Read the model definition and answer for the solid it produces. Units are mm, in the model's axes. A direction names the side the tool comes from. Coordinates: 2 decimals unless noted, no trailing zeros. Order: outer loops, then holes, each group sorted by start corner. A loop starts at its lowest first (then second) coordinate and runs counter-clockwise, first axis right, second up. Notation, with made-up numbers: (79.5, -5.5) -> (122.5, -5.5) arc R20 ccw to (122.5, 23.5) -> close; hole circle Ø7 at (-17.75, -12.75). An arc over 180 degrees is marked (long way). Answer as a JSON object with one key per item and string values. Group by question number.
1) A tool of negligible diameter and unlimited length cuts with its end or side. For faces 1 (the flat face through (-34, -4, 17.8)), 2 (the flat face through (-9, 66, 17.8)), 3 (the flat face through (18.9, 40, 17)), from which of +Z, -Z, +X, -X, +Y, -Y can it reach the whole face along a straight path? Write none if from no direction.
2) Section C-C on y = 53.5 is taken. Determine the outline of the cut face in (x, z).
3) Consider L1, parallel to X at y = 5, z = 16.8; L2, parallel to Y at x = -53, z = 18.5; L3, parallel to Y at x = -33, z = 18.7. Determine where each line is inside the solid, lowest interval first.
4) Section D-D on x = 46 is taken. Determine the outline of the cut face in (y, z), and give its area (3 significant figures).
5) Section B-B on x = -24.13 is taken. Determine the outline of the cut face in (y, z), and give its area (3 significant figures).
6) Determine the mould class of faces 4 (the flat face through (14.53, 37.6, 17.48)), 5 (the flat face through (25, 65, 17)) for opening direction X: released by +X, released by -X, zero draft, split by the parting line, or undercut.
7) Given pin 1 (1.5 mm diameter, centred on x = -23, y = 11.5, fed in from -Z); pin 2 (0.9 mm diameter, centred on y = 40.5, z = 17.5, fed in from -X); pin 3 (1.4 mm diameter, centred on x = 33, y = -3, fed in from -Z); pin 4 (1.5 mm diameter, centred on x = 20.5, z = 18, fed in from +Y), each flat-ended and moving along its own axis, determine where each tip first touches the part or whether it passes through.
8) Section A-A on x = 2.7 is taken. Determine the outline of the cut face in (y, z), and give its area (3 significant figures).
from build123d import *

# Parameters (mm, degrees)
PAD001_DEPTH         = 3
SKETCH012_R          = 1.4
POCKET005_DEPTH      = 3.001
SKETCH014_R          = 2.5
POCKET006_DEPTH      = 1.8
POCKET008_DEPTH      = 0.001
POCKET008_DEPTH_BACK = 3.001
SKETCH017_R          = 1.15
POCKET009_DEPTH      = 0.001
POCKET009_DEPTH_BACK = 3.001
POCKET010_DEPTH      = 1.8
SKETCH023_R          = 1.15
POCKET013_DEPTH      = 0.001
POCKET013_DEPTH_BACK = 3.001
SKETCH026_R          = 2.15
POCKET016_DEPTH      = 2.001


with BuildPart() as part:
    # Sketch009 → Pad001 (new body)
    with BuildSketch(Plane.XY):
        with BuildLine():
            Line((56.5, 38), (56.5, -1))
            ThreePointArc((54.5, -3), (55.914214, -2.414214), (56.5, -1))
            Line((54.5, -3), (30.5, -3))
            ThreePointArc((29.5, -2), (29.792893, -2.707107), (30.5, -3))
            Line((29.5, -2), (29.5, -1))
            ThreePointArc((29.5, -1), (29.207107, -0.292893), (28.5, 0))
            Line((28.5, 0), (-28.5, 0))
            ThreePointArc((-28.5, 0), (-29.207107, -0.292893), (-29.5, -1))
            Line((-29.5, -1), (-29.5, -2))
            ThreePointArc((-30.5, -3), (-29.792893, -2.707107), (-29.5, -2))
            Line((-30.5, -3), (-54.5, -3))
            ThreePointArc((-56.5, -1), (-55.914214, -2.414214), (-54.5, -3))
            Line((-56.5, -1), (-56.5, 38))
            ThreePointArc((-54.500018, 40), (-55.91422, 39.414207), (-56.5, 38))
            Line((-54.500018, 40), (-38, 40))
            ThreePointArc((-38, 40), (-36.585786, 40.585786), (-36, 42))
            Line((-36, 67), (-36, 42))
            ThreePointArc((-34, 69), (-35.414214, 68.414214), (-36, 67))
            Line((-34, 69), (-15.656854, 69))
            ThreePointArc((-15.656854, 69), (-14.891487, 69.152241), (-14.242641, 69.585786))
            Line((-14.242641, 69.585786), (-7.414214, 76.414214))
            ThreePointArc((-6, 77), (-6.765367, 76.847759), (-7.414214, 76.414214))
            Line((-6, 77), (6, 77))
            ThreePointArc((7.414214, 76.414214), (6.765367, 76.847759), (6, 77))
            Line((7.414214, 76.414214), (14.242641, 69.585786))
            ThreePointArc((14.242641, 69.585786), (14.891487, 69.152241), (15.656854, 69))
            Line((15.656854, 69), (34, 69))
            ThreePointArc((36, 67), (35.414214, 68.414214), (34, 69))
            Line((36, 42), (36, 67))
            ThreePointArc((36, 42), (36.585786, 40.585786), (38, 40))
            Line((38, 40), (54.500018, 40))
            ThreePointArc((56.5, 38), (55.91422, 39.414207), (54.500018, 40))
        make_face()
    extrude(amount=PAD001_DEPTH)

    # Sketch012 → Pocket005 (cut, through all)
    with BuildSketch(Plane.XY):
        with Locations((-8.89, 66.04)):
            Circle(SKETCH012_R)
        with Locations((19.05, 66.04)):
            Circle(SKETCH012_R)
        with Locations((24.13, 13.97)):
            Circle(SKETCH012_R)
        with Locations((-24.13, 15.24)):
            Circle(SKETCH012_R)
    extrude(amount=POCKET005_DEPTH, mode=Mode.SUBTRACT)

    # Sketch014 → Pocket006 (cut)
    with BuildSketch(Plane.XY):
        with Locations((-24.13, 15.24)):
            Circle(SKETCH014_R)
        with Locations((24.13, 13.97)):
            Circle(SKETCH014_R)
        with BuildLine():
            ThreePointArc((-11.39, 66.04), (-8.89, 63.54), (-6.39, 66.04))
            Line((-6.39, 66.04), (-6.39, 86.04))
            ThreePointArc((-6.39, 86.04), (-8.89, 88.54), (-11.39, 86.04))
            Line((-11.39, 66.04), (-11.39, 86.04))
        make_face()
        with BuildLine():
            ThreePointArc((16.55, 66.04), (19.05, 63.54), (21.55, 66.04))
            Line((21.55, 66.04), (21.55, 86.04))
            ThreePointArc((21.55, 86.04), (19.05, 88.54), (16.55, 86.04))
            Line((16.55, 66.04), (16.55, 86.04))
        make_face()
    extrude(amount=POCKET006_DEPTH, mode=Mode.SUBTRACT)

    # Sketch015 → Pocket008 (cut, two sides)
    with BuildSketch(Plane.XY) as pocket008_sk:
        Polygon((-18.9, 45.774316), (-18.9, 42.425684), (-16, 40.751368), (-13.1, 42.425684), (-13.1, 45.774316), (-16, 47.448632), align=None)
        Polygon((13.1, 45.774316), (13.1, 42.425684), (16, 40.751368), (18.9, 42.425684), (18.9, 45.774316), (16, 47.448632), align=None)
        Polygon((-18.9, 31.574316), (-18.9, 28.225684), (-16, 26.551368), (-13.1, 28.225684), (-13.1, 31.574316), (-16, 33.248632), align=None)
        Polygon((13.1, 31.574316), (13.1, 28.225684), (16, 26.551368), (18.9, 28.225684), (18.9, 31.574316), (16, 33.248632), align=None)
    extrude(amount=-POCKET008_DEPTH, mode=Mode.SUBTRACT)
    extrude(pocket008_sk.sketch, amount=POCKET008_DEPTH_BACK, mode=Mode.SUBTRACT)

    # Sketch017 → Pocket009 (cut, two sides)
    with BuildSketch(Plane.XY) as pocket009_sk:
        with Locations((-53, 36)):
            Circle(SKETCH017_R)
        with Locations((-33, 1)):
            Circle(SKETCH017_R)
        with Locations((-53, 1)):
            Circle(SKETCH017_R)
        with Locations((53, 36)):
            Circle(SKETCH017_R)
        with Locations((53, 1)):
            Circle(SKETCH017_R)
        with Locations((33, 1)):
            Circle(SKETCH017_R)
    extrude(amount=-POCKET009_DEPTH, mode=Mode.SUBTRACT)
    extrude(pocket009_sk.sketch, amount=POCKET009_DEPTH_BACK, mode=Mode.SUBTRACT)

    # Sketch018 → Pocket010 (cut)
    with BuildSketch(Plane.XY):
        Polygon((53, 33.575129), (55.1, 34.787564), (55.1, 37.212436), (53, 38.424871), (50.9, 37.212436), (50.9, 34.787564), align=None)
        Polygon((53, 3.424871), (50.9, 2.212436), (50.9, -0.212436), (53, -1.424871), (55.1, -0.212436), (55.1, 2.212436), align=None)
        Polygon((33, 3.424871), (30.9, 2.212436), (30.9, -0.212436), (33, -1.424871), (35.1, -0.212436), (35.1, 2.212436), align=None)
        Polygon((-33, 3.424871), (-35.1, 2.212436), (-35.1, -0.212436), (-33, -1.424871), (-30.9, -0.212436), (-30.9, 2.212436), align=None)
        Polygon((-53, 3.424871), (-55.1, 2.212436), (-55.1, -0.212436), (-53, -1.424871), (-50.9, -0.212436), (-50.9, 2.212436), align=None)
        Polygon((-53, 33.575129), (-50.9, 34.787564), (-50.9, 37.212436), (-53, 38.424871), (-55.1, 37.212436), (-55.1, 34.787564), align=None)
    extrude(amount=POCKET010_DEPTH, mode=Mode.SUBTRACT)

    # Sketch023 → Pocket013 (cut, two sides)
    with BuildSketch(Plane.XY) as pocket013_sk:
        with Locations((-40, 9)):
            Circle(SKETCH023_R)
        with Locations((40, 9)):
            Circle(SKETCH023_R)
        with Locations((2.7, 72.5)):
            Circle(SKETCH023_R)
        with Locations((-2.7, 72.5)):
            Circle(SKETCH023_R)
    extrude(amount=-POCKET013_DEPTH, mode=Mode.SUBTRACT)
    extrude(pocket013_sk.sketch, amount=POCKET013_DEPTH_BACK, mode=Mode.SUBTRACT)

    # Sketch026 (on DatumPlane) → Pocket016 (cut, through all)
    with BuildSketch(Plane.XY.offset(1)):
        with Locations((-40, 9)):
            Circle(SKETCH026_R)
        with Locations((40, 9)):
            Circle(SKETCH026_R)
    extrude(amount=POCKET016_DEPTH, mode=Mode.SUBTRACT)


with BuildPart() as part_1:
    # Body001 placement: moved
    add(part.part.moved(Location((0, -4, 16))))


solid = part_1.part
Worked answers:
{
 "1": {"face 1": "-Z", "face 2": "-Z, +Y", "face 3": "+Z, -Z"},
 "2": {"outline": "(-36, 16) -> (36, 16) -> (36, 19) -> (-36, 19) -> close"},
 "3": {"L1": "x = -56.5 to -41.15, -38.85 to 38.85, 41.15 to 56.5", "L2": "y = -7 to -4.15, -1.85 to 30.85, 33.15 to 36", "L3": "y = -7 to -4.15, -1.85 to 65"},
 "4": {"outline": "(-7, 16) -> (36, 16) -> (36, 19) -> (-7, 19) -> close", "area": "129 mm²"},
 "5": {"outline": "(-4, 16) -> (8.74, 16) -> (8.74, 17.8) -> (9.84, 17.8) -> (9.84, 19) -> (-4, 19) -> close; (12.64, 17.8) -> (13.74, 17.8) -> (13.74, 16) -> (65, 16) -> (65, 19) -> (12.64, 19) -> close", "area": "195 mm²"},
 "6": {"face 4": "undercut", "face 5": "zero draft"},
 "7": {"pin 1": "stops at z = 17.8", "pin 2": "stops at x = -36", "pin 3": "passes through", "pin 4": "stops at y = 65"},
 "8": {"outline": "(-4, 16) -> (67.35, 16) -> (67.35, 19) -> (-4, 19) -> close; (69.65, 16) -> (73, 16) -> (73, 19) -> (69.65, 19) -> close", "area": "224 mm²"}
}
